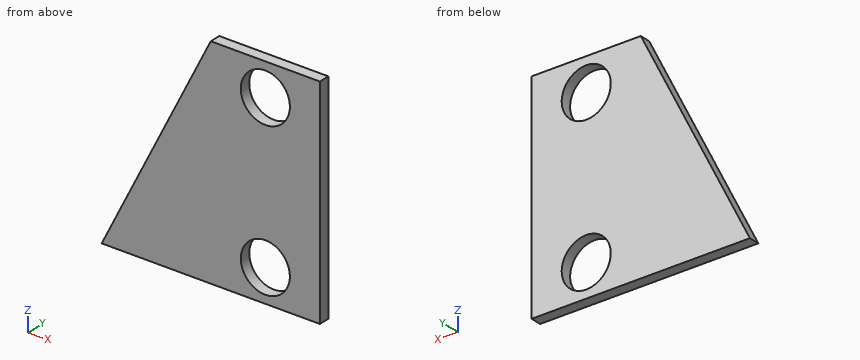
from build123d import *

# Parameters (mm, degrees)
SKETCH1_R           = 2.25
BOSS_EXTRUDE1_DEPTH = 1


with BuildPart() as part:
    # Sketch1 → Boss-Extrude1 (new body)
    with BuildSketch(Plane(origin=(0, 0, 0), x_dir=(1, 0, 0), z_dir=(0, 1, 0))):
        Polygon((-5, -10), (-15, 10), (-5, 10), (5, 10), (5, -10), align=None)
        with Locations(Location((0, 7, 0), (0, 0, 270))):
            Circle(SKETCH1_R, mode=Mode.SUBTRACT)
        with Locations(Location((0, -7, 0), (0, 0, 270))):
            Circle(SKETCH1_R, mode=Mode.SUBTRACT)
    extrude(amount=BOSS_EXTRUDE1_DEPTH)


solid = part.part
The listing builds one solid part. Answer for the finished solid, in the listing's coordinates (mm). Give positions to 0.01 mm unless a question says otherwise; leave off trailing zeros. Order: outer loops, then holes, each group sorted by start corner. A loop starts at its lowest first (then second) coordinate and runs counter-clockwise, first axis right, second up. Notation, with made-up numbers: (50, 49.5) - (70, 49.5) arc R9 ccw to (70, 59.5) - close; hole circle Ø4 at (-18, 74.5). An arc over 180 degrees is marked (long way). One line per item, written item: value. Start each with the question number.
1) A cutting plane is placed at C-C on y = 0.65. Give the vertices of the cut face in (x, z), then the cut area to 3 significant figures.
2) A cutting plane is placed at D-D on z = 7. Give the vertices of the cut face in (x, y), then the cut area to 3 significant figures.
3) Find the intervals of material crossed by L1, parallel to Z at x = 1.25, y = 0.9; L2, parallel to Z at x = 2, y = 0.4; L3, parallel to X at y = 0.65, z = 7, in increasing order.
4) A cutting plane is placed at A-A on z = -7. Give the vertices of the cut face in (x, y), then the cut area to 3 significant figures.
5) A cutting plane is placed at B-B on x = 0. Give the vertices of the cut face in (y, z).
6) Given pin 1 Ø2.5 at (x, z) = (0, 7) entering from +Y, flat-ended and moving along its own axis, determine where the tip first touches the part or whether it passes through.
Answer sheet:
1. outline: (-15, -10) - (5, -10) - (5, 10) - (-5, 10) - close; hole circle Ø4.5 at (0, -7); hole circle Ø4.5 at (0, 7)
1. area: 268 mm2
2. outline: (-6.5, 0) - (-2.25, 0) - (-2.25, 1) - (-6.5, 1) - close; (2.25, 0) - (5, 0) - (5, 1) - (2.25, 1) - close
2. area: 7.00 mm2
3. L1: z = -10 to -8.87, -5.13 to 5.13, 8.87 to 10
3. L2: z = -10 to -8.03, -5.97 to 5.97, 8.03 to 10
3. L3: x = -6.5 to -2.25, 2.25 to 5
4. outline: (-13.5, 0) - (-2.25, 0) - (-2.25, 1) - (-13.5, 1) - close; (2.25, 0) - (5, 0) - (5, 1) - (2.25, 1) - close
4. area: 14.0 mm2
5. outline: (0, -10) - (1, -10) - (1, -9.25) - (0, -9.25) - close; (0, -4.75) - (1, -4.75) - (1, 4.75) - (0, 4.75) - close; (0, 9.25) - (1, 9.25) - (1, 10) - (0, 10) - close
6. pin 1: passes through
